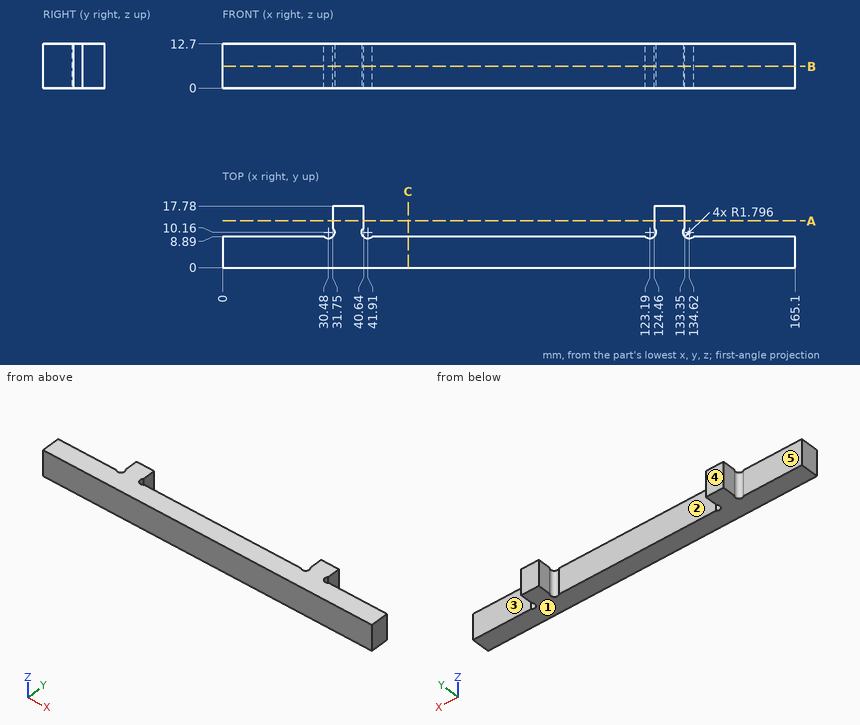
Can you work these out from the drawing? Everything is in mm from the part's minimum corner. A direction names the side the tool comes from. Coordinates: 2 decimals unless noted, no trailing zeros. Loops run counter-clockwise (first coordinate to the right, second up) from the corner with the lowest first, then second, coordinate; pieces in that order, holes last. Notation, with made-up numbers: M 32,14.25 L 37,14.25 A32 ccw 37,52.25 Z; hole C 44,82 d2. An arc over 180 degrees is marked long. Put each result on its own line as item: value. Start each with the question number.
(1) Suppose I cut it at B-B on z = 6.25. Please give me the cut outline in (x, y), then the cut area to 3 significant figures.
(2) Will these pins go through, and if not, where does the flat tip stop? P1, Ø1.9, axis at y = 14, z = 7, coming from the +X side; P2, Ø6.5, axis at x = 97.5, z = 7, coming from the +Y side; P3, Ø3, axis at y = 13, z = 5, coming from the -X side.
(3) Suppose I cut it at A-A on y = 13.5. Please give me the cut outline in (x, z), then the cut area to 3 significant figures.
(4) I need wall thicknesses on line 1 (X direction, y = 13.5, z = 10.25); line 2 (Y direction, x = 52, z = 4.75); line 3 (X direction, y = 9.25, z = 10.75). Which ranges of each line are inside material? Lowest first, please. Write a range as from..to.
(5) Thinking about a two-plate mould opening in X: for the marked faces 1 and 2, which applies, pulls with the +X half, pulls with the -X half, needs draft (parallel to the pull), parting line crosses it, or undercut?
(6) Suppose I cut it at C-C on x = 53.5. Please give me the cut outline in (y, z), then the cut area to 3 significant figures.
(7) For the marked faces 3, 4 and 5, which set-ups out of +Z, -Z, +X, -X, +Y, -Y let a thin tool reach every point of the face, with its end or its side?
Solutions:
1. outline: M 0,0 L 165.1,0 L 165.1,8.89 L 135.89,8.89 A1.8 cw 133.35,11.43 L 133.35,17.78 L 124.46,17.78 L 124.46,11.43 A1.8 cw 121.92,8.89 L 43.18,8.89 A1.8 cw 40.64,11.43 L 40.64,17.78 L 31.75,17.78 L 31.75,11.43 A1.8 cw 29.21,8.89 L 0,8.89 Z
1. area: 1,620 mm2
2. P1: stops at x = 133.35
2. P2: stops at y = 8.89
2. P3: stops at x = 31.75
3. outline: M 31.75,0 L 40.64,0 L 40.64,12.7 L 31.75,12.7 Z; M 124.46,0 L 133.35,0 L 133.35,12.7 L 124.46,12.7 Z
3. area: 226 mm2
4. line 1: x = 31.75..40.64, 124.46..133.35
4. line 2: y = 0..8.89
4. line 3: x = 32.03..40.36, 124.74..133.07
5. face 1: needs draft
5. face 2: undercut
6. outline: M 0,0 L 8.89,0 L 8.89,12.7 L 0,12.7 Z
6. area: 113 mm2
7. face 3: +Z, -Z, +X, +Y
7. face 4: +Z, -Z, +X, -X, +Y
7. face 5: +Z, -Z, -X, +Y
